Can you work these out from the model? Positions are in its coordinate system, mm. A direction names the side the tool comes from. Give positions to 0.01 mm unless a question says otherwise; leave off trailing zeros. Loops run counter-clockwise (first coordinate to the right, second up) from the corner with the lowest first, then second, coordinate; pieces in that order, holes last. Notation, with made-up numbers: (-34, 9) - (-20, 9) arc R26 ccw to (-20, 45) - close; hole circle Ø2 at (50, -23). An arc over 180 degrees is marked (long way). Answer as a JSON object with one key per item and string values. Group by question number.
Item 1: Which directions (+Z, -Z, +X, -X, +Y, -Y) give clear straight access to the entire face, cutting with the end or side of a thin tool? Please do faces 1 (the flat face through (-0.2, 15, -8.4)), 2 (the flat face through (4.5, 7, 1)).
Item 2: Thinking about a two-plate mould opening in X: for faces 3 (the flat face through (7, 10.5, 1)), 4 (the flat face through (8, 4, 0)), 5 (the flat face through (0, 7, -14)), which applies, pulls with the +X half, pulls with the -X half, needs draft (parallel to the pull), parting line crosses it, or undercut?
Item 3: Suppose I cut it at B-B on x = 9. Write out the boundary of the cut face in (y, z).
Item 4: Suppose I cut it at C-C on y = 1.5. Write out the boundary of the cut face in (x, z), and give its area (3 significant figures).
Item 5: Will these pins go through, and if not, where does the flat tip stop? pin 1 (4 mm diameter, centred on x = 4, y = 5.5, fed in from -Z); pin 2 (1.6 mm diameter, centred on y = 7, z = 0.5, fed in from +X).
Item 6: Suppose I cut it at A-A on y = 8.5. Write out the boundary of the cut face in (x, z), and give its area (3 significant figures).
Item 7: Please list where these lines run through material, in increasing order: L1, parallel to X at y = 9.25, z = -10.25; L2, parallel to Z at x = 9, y = 13.75; L3, parallel to Z at x = -0.5, y = 12.
Item 8: Suppose I cut it at D-D on z = -1. Write out the boundary of the cut face in (x, y), and give its area (3 significant figures).
from build123d import *

# Parameters (mm, degrees)
EXTRUDE_1_DEPTH     = 15
SKETCH_2_W          = 6
SKETCH_2_H          = 6
CUT_EXTRUDE_1_DEPTH = 38.436613095


with BuildPart() as part:
    # Эскиз1 → Бобышка-Вытянуть1 (new body)
    with BuildSketch(Plane(origin=(0, 0, 0), x_dir=(1, 0, 0), z_dir=(0, 1, 0))):
        Polygon((-2, 25.5), (-2, -2), (17.5, -2), (15.5, 0), (0, 0), (0, 27.5), align=None)
    extrude(amount=EXTRUDE_1_DEPTH)

    # Эскиз2 → Вырез-Вытянуть1 (cut, through all)
    with BuildSketch(Plane.XY.offset(2)):
        with Locations((7.5, 7.5)):
            Rectangle(SKETCH_2_W, SKETCH_2_H)
    extrude(amount=-CUT_EXTRUDE_1_DEPTH, mode=Mode.SUBTRACT)


solid = part.part
Worked out:
{
 "1": {"face 1": "+Z, -Z, +X, -X, +Y", "face 2": "+Z, -Z"},
 "2": {"face 3": "undercut", "face 4": "needs draft", "face 5": "pulls with the +X half"},
 "3": {"outline": "(0, 0) - (4.5, 0) - (4.5, 2) - (0, 2) - close; (10.5, 0) - (15, 0) - (15, 2) - (10.5, 2) - close"},
 "4": {"outline": "(-2, -25.5) - (0, -27.5) - (0, 0) - (15.5, 0) - (17.5, 2) - (-2, 2) - close", "area": "90.0 mm2"},
 "5": {"pin 1": "stops at z = 0", "pin 2": "stops at x = 16.8"},
 "6": {"outline": "(-2, -25.5) - (0, -27.5) - (0, 0) - (4.5, 0) - (4.5, 2) - (-2, 2) - close; (10.5, 0) - (15.5, 0) - (17.5, 2) - (10.5, 2) - close", "area": "78.0 mm2"},
 "7": {"L1": "x = -2 to 0", "L2": "z = 0 to 2", "L3": "z = -27 to 2"},
 "8": {"outline": "(-2, 0) - (0, 0) - (0, 15) - (-2, 15) - close", "area": "30.0 mm2"}
}
